```python
from build123d import *

# Parameters (mm, degrees)
SKETCH1_W                      = 305
SKETCH1_H                      = 327
BOSS_EXTRUDE1_DEPTH            = 6.35
CUT_EXTRUDE1_DEPTH             = 7.35
SKETCH3_W                      = 10
SKETCH3_H                      = 6.35
BOSS_EXTRUDE2_DEPTH            = 19
SKETCH4_W                      = 253
SKETCH4_H                      = 16
CUT_EXTRUDE2_DEPTH             = 7.35
DRAFT1_ANGLE                   = 45
F_4_3_4_3_DIAMETER_HOLE1_D     = 4.3
F_2_5_2_5_DIAMETER_HOLE1_D     = 2.5
F_2_5_2_5_DIAMETER_HOLE1_DEPTH = 6.35
CHAMFER1_SIZE                  = 2.55
FILLET1_R                      = 3
FILLET2_R                      = 5
FILLET3_R                      = 15


with BuildPart() as part:
    # Sketch1 → Boss-Extrude1 (new body)
    with BuildSketch(Plane(origin=(0, 6.35, 0), x_dir=(1, 0, 0), z_dir=(0, 1, 0))):
        with Locations((0, -5)):
            Rectangle(SKETCH1_W, SKETCH1_H)
    extrude(amount=-BOSS_EXTRUDE1_DEPTH)

    # Sketch2 → Cut-Extrude1 (cut, through all)
    with BuildSketch(Plane(origin=(0, 6.35, 0), x_dir=(-1, 0, 0), z_dir=(0, 1, 0))):
        with BuildLine():
            Line((-143.448007721, -158.5), (143.448007721, -158.5))
            ThreePointArc((143.448007721, -158.5), (140.601020514, -154.17544468), (135.702041029, -152.5))
            Line((135.702041029, -152.5), (-135.702041029, -152.5))
            ThreePointArc((-135.702041029, -152.5), (-140.601020514, -154.17544468), (-143.448007721, -158.5))
        make_face()
    extrude(amount=-CUT_EXTRUDE1_DEPTH, mode=Mode.SUBTRACT)

    # Sketch3 → Boss-Extrude2 (add)
    with BuildSketch(Plane(origin=(0, 0, -152.5), x_dir=(-1, 0, 0), z_dir=(0, 0, -1))):
        with Locations((0, 3.175)):
            Rectangle(SKETCH3_W, SKETCH3_H)
    extrude(amount=BOSS_EXTRUDE2_DEPTH)

    # Sketch4 → Cut-Extrude2 (cut, through all)
    with BuildSketch(Plane.XZ):
        with Locations((0, 160.5)):
            Rectangle(SKETCH4_W, SKETCH4_H)
    extrude(amount=-CUT_EXTRUDE2_DEPTH, mode=Mode.SUBTRACT)

    # Draft1
    draft1_faces = [part.faces().sort_by_distance(p)[0] for p in [
        (-126.5, 3.175, 160.5),
        (126.5, 3.175, 160.5),
    ]]
    draft(draft1_faces, Plane(origin=(-126.5, 6.35, 152.5), x_dir=(1, 0, 0), z_dir=(0, 0, 1)), DRAFT1_ANGLE)

    # Ø4.3 (4.3) Diameter Hole1 (through all)
    with Locations(Plane(origin=(0, 6.35, 0), x_dir=(1, 0, 0), z_dir=(0, 1, 0))):
        with Locations((0, 166.5), (-147.5, -163.5), (147.5, -163.5)):
            Hole(F_4_3_4_3_DIAMETER_HOLE1_D / 2)

    # Ø2.5 (2.5) Diameter Hole1
    with Locations(Plane(origin=(0, 0, 0), x_dir=(-1, 0, 0), z_dir=(0, -1, 0))):
        with Locations((147.5, 154), (-147.5, 154), (-137.107695155, -157.5), (137.107695155, -157.5), (0, 155.5)):
            Hole(F_2_5_2_5_DIAMETER_HOLE1_D / 2, depth=F_2_5_2_5_DIAMETER_HOLE1_DEPTH)

    # Chamfer1
    chamfer1_edges = [part.edges().sort_by_distance(p)[0] for p in [
        (149.65, 6.35, 163.5),
        (-145.35, 6.35, 163.5),
        (2.15, 6.35, -166.5),
    ]]
    chamfer(chamfer1_edges, length=CHAMFER1_SIZE)

    # Fillet1
    fillet1_edges = [part.edges().sort_by_distance(p)[0] for p in [
        (143.448007721, 3.175, -158.5),
        (-143.448007721, 3.175, -158.5),
        (-5, 3.175, -171.5),
        (5, 3.175, -171.5),
        (-152.5, 3.175, -158.5),
        (152.5, 3.175, -158.5),
    ]]
    fillet(fillet1_edges, radius=FILLET1_R)

    # Fillet2
    fillet2_edges = [part.edges().sort_by_distance(p)[0] for p in [
        (-142.5, 3.175, 168.5),
        (142.5, 3.175, 168.5),
        (152.5, 3.175, 168.5),
        (-152.5, 3.175, 168.5),
    ]]
    fillet(fillet2_edges, radius=FILLET2_R)

    # Fillet3
    fillet3_edges = [part.edges().sort_by_distance(p)[0] for p in [
        (-5, 3.175, -152.5),
        (5, 3.175, -152.5),
        (126.5, 3.175, 152.5),
        (-126.5, 3.175, 152.5),
    ]]
    fillet(fillet3_edges, radius=FILLET3_R)


solid = part.part
```
Verification items for the finished model (mm, model axes). A direction names the side the tool comes from. Give positions to 0.01 mm unless a question says otherwise; leave off trailing zeros. Loops run counter-clockwise (first coordinate to the right, second up) from the corner with the lowest first, then second, coordinate; pieces in that order, holes last. Notation, with made-up numbers: M 59,87.25 L 112,87.25 A16 cw 112,108.25 Z; hole C 46.5,58 d8. An arc over 180 degrees is marked long. One line per question, with ' | ' between items.
Item 1: Section check B-B, the plane x = 73. Record the cut outline in (y, z), plus the area to 3 significant figures.
Completed:
outline: M 0,-152.5 L 6.35,-152.5 L 6.35,152.5 L 0,152.5 Z | area: 1,940 mm^2
Item 2: Draft check along Z on faces 4 (the face through (-2, 0, -4)), 5 (the face through (136, 3, 162)), 6 (the face through (-9.51, 3.22, -156.78)), 7 (the face through (0.3, 3.92, -168.75)). Enter one of: +Z half, -Z half, draft (parallel to the pull), parting line (faces both ways), or undercut.
Completed:
face 4: draft | face 5: +Z half | face 6: -Z half | face 7: undercut
Item 3: Section check A-A, the plane y = 1. State how many separate pieces and enclosed holes the cut face has, plus the area to 3 significant figures.
Completed:
separate pieces: 1 | enclosed holes: 8 | area: 93,900 mm^2
Item 4: Depth check by flat-ended pin: P1, Ø1.5, axis at x = -89, y = 3.5, coming from the +Z side; P2, Ø0.5, axis at y = 3.5, z = -168, coming from the -X side; P3, Ø7, axis at x = -147.5, z = 163.5, coming from the +Y side; P4, Ø1.5, axis at x = 137.11, z = 157.5, coming from the -Y side. Enter the tip coordinate at first touch or a pass-through.
Completed:
P1: stops at z = 152.5 | P2: stops at x = -5 | P3: stops at y = 5.15 | P4: passes through
Item 5: Tool access check on faces 1 (the face through (-136, 3, 162)), 2 (the face through (-145.7, 3.92, 164.88)), 3 (the face through (9.28, 3.22, -157.01)). Record the directions out of +Z, -Z, +X, -X, +Y, -Y that give a thin tool (end or side, any length) a straight path to the whole face; none if there is none.
Completed:
face 1: +Z, +Y, -Y | face 2: +Y | face 3: -Z, +Y, -Y
Item 6: Thickness scan on line 1 (Z direction, x = -147.5, y = 2.25); line 2 (X direction, y = 1.75, z = 157.5); line 3 (Z direction, x = 1, y = 1.75). Record the ranges inside material, lowest first. Write a range as [from, to].
Completed:
line 1: z = [-158.5, -155.25], [-152.75, 161.35], [165.65, 168.5] | line 2: x = [-152.5, -138.36], [-135.86, -131.5], [131.5, 135.86], [138.36, 152.5] | line 3: z = [-171.5, -168.4], [-164.6, -156.25], [-154.75, 152.5]
